```python
from build123d import *

# Parameters (mm, degrees)
SKETCH1_W           = 355.6
SKETCH1_H           = 58.42
BOSS_EXTRUDE1_DEPTH = 4.7625
BOSS_EXTRUDE2_DEPTH = 4.7625
FILLET1_R           = 3.175
SKETCH3_W           = 6.858
SKETCH3_H           = 21.806929344
SKETCH3_W_2         = 6.35
SKETCH3_H_2         = 21.298929344
CUT_EXTRUDE1_DEPTH  = 209.73467472
SKETCH4_W           = 1.5875
SKETCH4_H           = 18.796
CUT_EXTRUDE2_DEPTH  = 209.73467472
SKETCH5_W           = 1.5875
SKETCH5_H           = 28.002862447
CUT_EXTRUDE3_DEPTH  = 208.38411122
SKETCH6_W           = 0.3175
SKETCH6_H           = 21.806929344
BOSS_EXTRUDE3_DEPTH = 4.7625
SKETCH7_W           = 0.3175
SKETCH7_H           = 21.806929344
CUT_EXTRUDE4_DEPTH  = 208.38411122
SKETCH8_W           = 152.4
SKETCH8_H           = 17.145
CUT_EXTRUDE5_DEPTH  = 208.38411122
FILLET2_R           = 6.35


with BuildPart() as part:
    # Sketch1 → Boss-Extrude1 (new body)
    with BuildSketch(Plane(origin=(0, 0, 0), x_dir=(1, 0, 0), z_dir=(0, 1, 0))):
        Rectangle(SKETCH1_W, SKETCH1_H)
    extrude(amount=BOSS_EXTRUDE1_DEPTH)

    # Sketch2 → Boss-Extrude2 (add)
    with BuildSketch(Plane(origin=(0, 4.7625, 0), x_dir=(1, 0, 0), z_dir=(0, 1, 0))):
        Polygon((177.8, -29.21), (88.9, -109.245791791), (76.2, -109.245791791), (76.2, -29.21), align=None)
        Polygon((-177.8, -29.21), (-88.9, -109.245791791), (-76.2, -109.245791791), (-76.2, -29.21), align=None)
    extrude(amount=-BOSS_EXTRUDE2_DEPTH)

    # Fillet1
    fillet1_edges = [part.edges().sort_by_distance(p)[0] for p in [
        (-76.2, 2.38125, 29.21),
        (76.2, 2.38125, 29.21),
    ]]
    fillet(fillet1_edges, radius=FILLET1_R)

    # Sketch3 → Cut-Extrude1 (cut, through all)
    with BuildSketch(Plane(origin=(0, 0, 0), x_dir=(-1, 0, 0), z_dir=(0, -1, 0))):
        with Locations((-174.625, -0.489464672)):
            Rectangle(SKETCH3_W, SKETCH3_H)
        with Locations((-174.625, -0.489464672)):
            Rectangle(SKETCH3_W_2, SKETCH3_H_2, mode=Mode.SUBTRACT)
        with Locations((-79.375, -0.489464672)):
            Rectangle(SKETCH3_W, SKETCH3_H)
        with Locations((-79.375, -0.489464672)):
            Rectangle(SKETCH3_W_2, SKETCH3_H_2, mode=Mode.SUBTRACT)
        with Locations((-79.375, -70.339464672)):
            Rectangle(SKETCH3_W, SKETCH3_H)
        with Locations((-79.375, -70.339464672)):
            Rectangle(SKETCH3_W_2, SKETCH3_H_2, mode=Mode.SUBTRACT)
        with Locations((79.375, -70.339464672)):
            Rectangle(SKETCH3_W, SKETCH3_H)
        with Locations((79.375, -70.339464672)):
            Rectangle(SKETCH3_W_2, SKETCH3_H_2, mode=Mode.SUBTRACT)
        with Locations((79.375, -0.489464672)):
            Rectangle(SKETCH3_W, SKETCH3_H)
        with Locations((79.375, -0.489464672)):
            Rectangle(SKETCH3_W_2, SKETCH3_H_2, mode=Mode.SUBTRACT)
        with Locations((174.625, -0.489464672)):
            Rectangle(SKETCH3_W, SKETCH3_H)
        with Locations((174.625, -0.489464672)):
            Rectangle(SKETCH3_W_2, SKETCH3_H_2, mode=Mode.SUBTRACT)
    extrude(amount=-CUT_EXTRUDE1_DEPTH, mode=Mode.SUBTRACT)


with BuildPart() as body_2:
    # of the pieces the cut leaves, the one that is kept (cut_extrude1_keep)
    add(part.part.solids().sort_by_distance((76.2, 0, 109.245791791))[0])

    # Sketch4 → Cut-Extrude2 (cut, through all)
    with BuildSketch(Plane(origin=(0, 4.7625, 0), x_dir=(1, 0, 0), z_dir=(0, 1, 0))):
        Polygon((177.8, -11.392929344), (176.2125, -11.392929344), (176.2125, -30.639210568), (177.8, -29.21), align=None)
        with Locations((177.00625, 19.812)):
            Rectangle(SKETCH4_W, SKETCH4_H)
        with Locations((-177.00625, 19.812)):
            Rectangle(SKETCH4_W, SKETCH4_H)
        Polygon((-176.2125, -30.639210568), (-176.2125, -11.392929344), (-177.8, -11.392929344), (-177.8, -29.21), align=None)
    extrude(amount=-CUT_EXTRUDE2_DEPTH, mode=Mode.SUBTRACT)

    # Sketch5 → Cut-Extrude3 (cut, through all)
    with BuildSketch(Plane(origin=(0, 4.7625, 0), x_dir=(1, 0, 0), z_dir=(0, 1, 0))):
        with Locations((-76.99375, -95.244360567)):
            Rectangle(SKETCH5_W, SKETCH5_H)
        with Locations((76.99375, -95.244360567)):
            Rectangle(SKETCH5_W, SKETCH5_H)
    extrude(amount=-CUT_EXTRUDE3_DEPTH, mode=Mode.SUBTRACT)

    # Sketch6 → Boss-Extrude3 (add)
    with BuildSketch(Plane.XZ):
        with Locations((-76.10475, 0.489464672)):
            Rectangle(SKETCH6_W, SKETCH6_H)
        with Locations((76.10475, 0.489464672)):
            Rectangle(SKETCH6_W, SKETCH6_H)
    extrude(amount=-BOSS_EXTRUDE3_DEPTH)

    # Sketch7 → Cut-Extrude4 (cut, through all)
    with BuildSketch(Plane.XZ):
        with Locations((-82.96275, 0.489464672)):
            Rectangle(SKETCH7_W, SKETCH7_H)
        with Locations((-82.96275, 70.339464672)):
            Rectangle(SKETCH7_W, SKETCH7_H)
        with Locations((82.96275, 70.339464672)):
            Rectangle(SKETCH7_W, SKETCH7_H)
        with Locations((82.96275, 0.489464672)):
            Rectangle(SKETCH7_W, SKETCH7_H)
    extrude(amount=-CUT_EXTRUDE4_DEPTH, mode=Mode.SUBTRACT)

    # Sketch8 → Cut-Extrude5 (cut, through all)
    with BuildSketch(Plane(origin=(0, 4.7625, 0), x_dir=(1, 0, 0), z_dir=(0, 1, 0))):
        with Locations((0, -23.8125)):
            Rectangle(SKETCH8_W, SKETCH8_H)
    extrude(amount=-CUT_EXTRUDE5_DEPTH, mode=Mode.SUBTRACT)

    # Fillet2
    fillet2_edges = [body_2.edges().sort_by_distance(p)[0] for p in [
        (76.2, 2.38125, 15.24),
        (-76.2, 2.38125, 15.24),
    ]]
    fillet(fillet2_edges, radius=FILLET2_R)


solid = body_2.part
```
Geometry check sheet. Reference: the model listing, model coordinates, mm. A direction names the side the tool comes from. Give positions to 0.01 mm unless a question says otherwise; leave off trailing zeros. Order: outer loops, then holes, each group sorted by start corner. A loop starts at its lowest first (then second) coordinate and runs counter-clockwise, first axis right, second up.
1. Section check A-A, the plane z = 0. Enter the section's corners in (x, y), and give its area (3 significant figures).
2. Section check D-D, the plane x = 37. Enter the section's corners in (y, z).
3. Access from +Z, -Z, +X, -X, +Y, -Y to the whole of each face (thin tool, end or side, straight path). Record for faces 1 (the face through (74.29, 2.35, 17.05)), 2 (the face through (-2, 4.762, 10)).
4. Section check C-C, the plane y = 0.95. Give the number of separate pieces and of enclosed holes in the cut face, and give its area (3 significant figures).
5. Thickness scan on L1, parallel to Z at x = 81, y = 1.75; L2, parallel to X at y = 1, z = 8; L3, parallel to X at y = 3.05, z = 21.5. Record the ranges inside material, lowest first.
6. Gauge pin test, flat ends, axial feed: pin 1 Ø1.4 at (x, y) = (-174.5, 3) entering from +Z; pin 2 Ø2.5 at (x, y) = (173.5, 2) entering from +Z; pin 3 Ø1.4 at (y, z) = (3, 1) entering from -X. Record the tip position at first contact, or that the pin passes through.
7. Release check for a two-part mould opening along X. For faces 3 (the face through (-74.39, 2.35, 17.15)), 4 (the face through (-133.17, 2.41, 69.39)), 5 (the face through (133.17, 2.41, 69.39)) record: pulls with the +X half, pulls with the -X half, needs draft (parallel to the pull), parting line crosses it, or undercut.
8. Section check B-B, the plane z = 25.5. Enter the section's corners in (x, y).
Values follow:
1. outline: (-171.2, 0) - (-83.12, 0) - (-83.12, 4.76) - (-171.2, 4.76) - close; (-76.26, 0) - (76.26, 0) - (76.26, 4.76) - (-76.26, 4.76) - close; (83.12, 0) - (171.2, 0) - (171.2, 4.76) - (83.12, 4.76) - close
1. area: 1,570 mm2
2. outline: (0, -29.21) - (4.76, -29.21) - (4.76, 15.24) - (0, 15.24) - close
3. face 1: +Z, +Y, -Y
3. face 2: +Z, -Z, +X, -X, +Y
4. separate pieces: 1
4. enclosed holes: 2
4. area: 26,700 mm2
5. L1: z = -29.21 to -10.41, 11.39 to 59.44, 81.24 to 109.25
5. L2: x = -171.2 to -83.12, -76.26 to 76.26, 83.12 to 171.2
5. L3: x = -176.21 to -76.2, 76.2 to 176.21
6. pin 1: stops at z = 32.81
6. pin 2: stops at z = 34.21
6. pin 3: stops at x = -171.2
7. face 3: undercut
7. face 4: pulls with the -X half
7. face 5: pulls with the +X half
8. outline: (-176.21, 0) - (-76.2, 0) - (-76.2, 4.76) - (-176.21, 4.76) - close; (76.2, 0) - (176.21, 0) - (176.21, 4.76) - (76.2, 4.76) - close
